Could you check a few things on this model? Use its own coordinates, in mm. A direction names the side the tool comes from. Coordinates: 2 decimals unless noted, no trailing zeros. Loops run counter-clockwise (first coordinate to the right, second up) from the corner with the lowest first, then second, coordinate; pieces in that order, holes last.
from build123d import *

# Parameters (mm, degrees)
SKETCH_1_R      = 1.5
EXTRUDE_1_DEPTH = 3.5
SKETCH_2_R      = 1.15
EXTRUDE_2_DEPTH = 0.6
SKETCH_3_R      = 1.5
EXTRUDE_3_DEPTH = 71.8
SKETCH_4_R      = 1.15
EXTRUDE_4_DEPTH = 0.6
SKETCH_5_R      = 1.5
EXTRUDE_5_DEPTH = 3.5


with BuildPart() as part:
    # 草图1 → 凸台-拉伸1 (new body)
    with BuildSketch(Plane.XY):
        Circle(SKETCH_1_R)
    extrude(amount=EXTRUDE_1_DEPTH)

    # 草图2 → 凸台-拉伸2 (add)
    with BuildSketch(Plane.XY.offset(3.5)):
        Circle(SKETCH_2_R)
    extrude(amount=EXTRUDE_2_DEPTH)

    # 草图3 → 凸台-拉伸3 (add)
    with BuildSketch(Plane.XY.offset(4.1)):
        Circle(SKETCH_3_R)
    extrude(amount=EXTRUDE_3_DEPTH)

    # 草图4 → 凸台-拉伸4 (add)
    with BuildSketch(Plane.XY.offset(75.9)):
        Circle(SKETCH_4_R)
    extrude(amount=EXTRUDE_4_DEPTH)

    # 草图5 → 凸台-拉伸5 (add)
    with BuildSketch(Plane.XY.offset(76.5)):
        Circle(SKETCH_5_R)
    extrude(amount=EXTRUDE_5_DEPTH)


solid = part.part
(1) Which directions (+Z, -Z, +X, -X, +Y, -Y) give clear straight access to the entire face, cutting with the end or side of a thin tool? Please do faces 1 (the face through (-0.91, -0.7, 76.2)), 2 (the face through (-1.5, 0.07, 39.5)).
Answers:
face 1: none
face 2: +Z, -Z
(2) We'd pull the mould along Z, two halves only. Please class faces 3 (the face through (0, 0, 0)), 4 (the face through (-0.91, -0.7, 3.8)), 5 (the face through (-1.5, 0.07, 1.73)): +Z half, -Z half, draft (parallel to the pull), parting line (faces both ways), or undercut.
Answers:
face 3: -Z half
face 4: undercut
face 5: draft
(3) I need wall thicknesses on probe 1 along Z at (x, y) = (-0.25, 1.3); probe 2 along X at (y, z) = (0.15, 12); probe 3 along Y at (x, z) = (1.3, 52.5). Which ranges of each line are inside material? Lowest first, please.
Answers:
probe 1: z = 0 to 3.5, 4.1 to 75.9, 76.5 to 80
probe 2: x = -1.49 to 1.49
probe 3: y = -0.75 to 0.75
(4) Imagine slicing it at B-B, the plane z = 74. Write out the boundary of the cut face in (x, y).
Answers:
outline: circle Ø3 at (0, 0)
(5) Imagine slicing it at A-A, the plane x = -0.55. Write out the boundary of the cut face in (y, z), and give its area (3 significant figures).
Answers:
outline: (-1.4, 0) - (1.4, 0) - (1.4, 3.5) - (1.01, 3.5) - (1.01, 4.1) - (1.4, 4.1) - (1.4, 75.9) - (1.01, 75.9) - (1.01, 76.5) - (1.4, 76.5) - (1.4, 80) - (-1.4, 80) - (-1.4, 76.5) - (-1.01, 76.5) - (-1.01, 75.9) - (-1.4, 75.9) - (-1.4, 4.1) - (-1.01, 4.1) - (-1.01, 3.5) - (-1.4, 3.5) - close
area: 222 mm2
(6) For pin 1 (1 mm diameter, centred on x = 1, z = 56, fed in from +Y); pin 2 (1 mm diameter, centred on y = 1, z = 71, fed in from -X), each with a flat end and sliding along its axis, tell me the tip position at first contact or that it passes through.
Answers:
pin 1: stops at y = 1.41
pin 2: stops at x = -1.41
